Job drawing, mm, ordinate dimensions from the low corner. One solid piece. A direction names the side the tool comes from. Give positions to 0.01 mm unless a question says otherwise; leave off trailing zeros. Loops run counter-clockwise (first coordinate to the right, second up) from the corner with the lowest first, then second, coordinate; pieces in that order, holes last. Notation, with made-up numbers: (77, -2.5) - (86, -2.5) arc R35 cw to (86, 31.5) - close; hole circle Ø9 at (-32.75, 31.25). An arc over 180 degrees is marked (long way). Use a Markdown table: item, result.
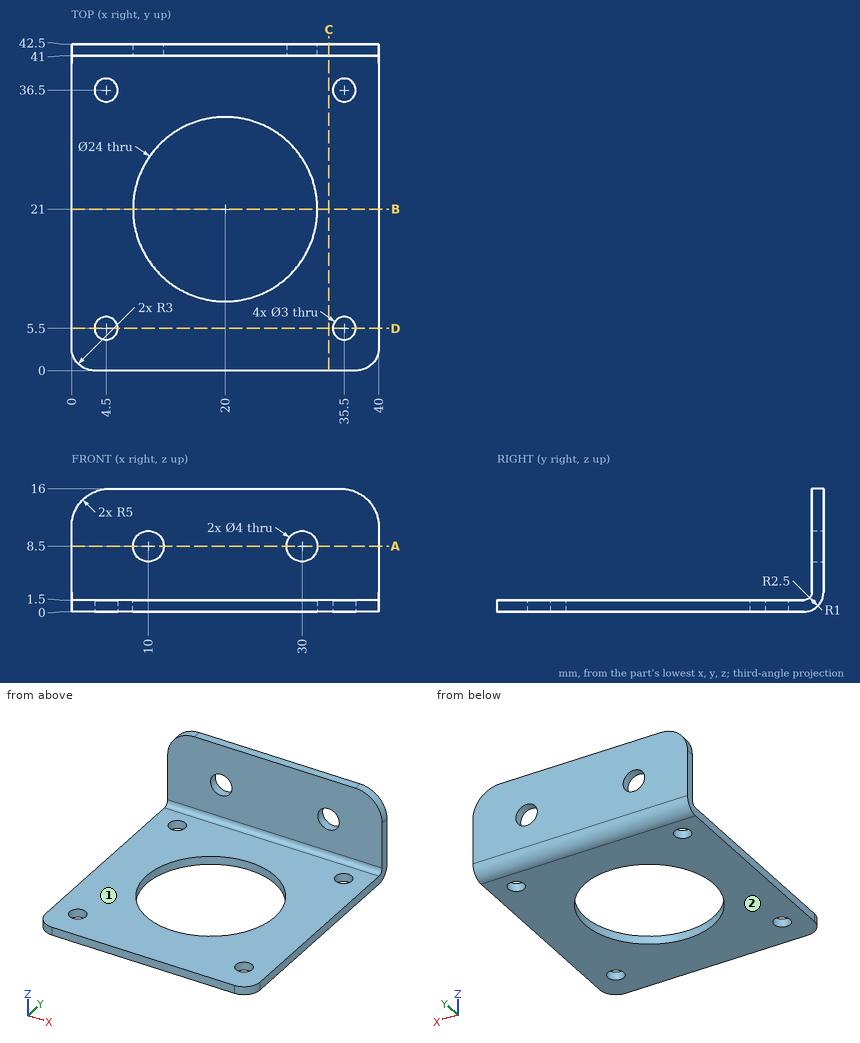
(1) Drill centre lines: probe 1 along Y at (x, z) = (4.5, 1); probe 2 along Y at (x, z) = (35.5, 0.65); probe 3 along Y at (x, z) = (8.5, 10). Where is each one in solid material? Low to high. Write a range as [from, to].
Computed:
| item | result |
|---|---|
| probe 1 | [0, 4], [7, 35], [38, 42] |
| probe 2 | [0, 4], [7, 35], [38, 41.68] |
| probe 3 | [41, 42.5] |
(2) Slice it at C-C, the plane x = 33.5. Write the cut outline in (y, z).
Computed:
| item | result |
|---|---|
| outline | (0, 0) - (40, 0) arc R2.5 ccw to (42.5, 2.5) - (42.5, 16) - (41, 16) - (41, 2.5) arc R1 cw to (40, 1.5) - (0, 1.5) - close |
(3) Slice it at A-A, the plane z = 8.5. Write the cut outline in (x, y).
Computed:
| item | result |
|---|---|
| outline | (0, 41) - (8, 41) - (8, 42.5) - (0, 42.5) - close; (12, 41) - (28, 41) - (28, 42.5) - (12, 42.5) - close; (32, 41) - (40, 41) - (40, 42.5) - (32, 42.5) - close |
(4) Slice it at B-B, the plane y = 21. Write the cut outline in (x, z).
Computed:
| item | result |
|---|---|
| outline | (0, 0) - (8, 0) - (8, 1.5) - (0, 1.5) - close; (32, 0) - (40, 0) - (40, 1.5) - (32, 1.5) - close |
(5) 3-axis set-ups, long thin cutter, end or side, ignore diameter. For the marked faces 1 and 2: which of +Z, -Z, +X, -X, +Y, -Y reach the whole face in a straight line?
Computed:
| item | result |
|---|---|
| face 1 | +Z, +X, -X, -Y |
| face 2 | -Z, +X, -X, +Y, -Y |
(6) Pin check, flat tips, straight feed: P1, Ø2, axis at x = 35, y = 18.5, coming from the +Z side; P2, Ø4.5, axis at x = 10, z = 8.5, coming from the -Y side. Stop position of each tip, or through.
Computed:
| item | result |
|---|---|
| P1 | z = 1.5 |
| P2 | y = 41 |
(7) Slice it at D-D, the plane y = 5.5. Write the cut outline in (x, z).
Computed:
| item | result |
|---|---|
| outline | (0, 0) - (3, 0) - (3, 1.5) - (0, 1.5) - close; (6, 0) - (34, 0) - (34, 1.5) - (6, 1.5) - close; (37, 0) - (40, 0) - (40, 1.5) - (37, 1.5) - close |
